Check sheet for the modelled part. Datum: model origin and axes. Units: mm. A direction names the side the tool comes from. Give positions to 0.01 mm unless a question says otherwise; leave off trailing zeros. Order: outer loops, then holes, each group sorted by start corner. A loop starts at its lowest first (then second) coordinate and runs counter-clockwise, first axis right, second up. Notation, with made-up numbers: M 89.25,24.5 L 100.25,24.5 A15 ccw 100.25,45.5 Z; hole C 87.5,-39.75 d9. An arc over 180 degrees is marked long. Return JSON: item names as keys, results as strings. Group by question number.
from build123d import *

# Parameters (mm, degrees)
SKETCH1_R           = 3
BOSS_EXTRUDE1_DEPTH = 3
CUT_EXTRUDE1_DEPTH  = 1.5
SKETCH4_R           = 1.35
BOSS_EXTRUDE2_DEPTH = 8.5


with BuildPart() as part:
    # Sketch1 → Boss-Extrude1 (new body)
    with BuildSketch(Plane.XY):
        Circle(SKETCH1_R)
    extrude(amount=BOSS_EXTRUDE1_DEPTH)

    # Sketch2 → Cut-Extrude1 (cut)
    with BuildSketch(Plane.XY.offset(3)):
        Polygon((2.06190779, 0), (1.030953895, 1.785664527), (-1.030953895, 1.785664527), (-2.06190779, 0), (-1.030953895, -1.785664527), (1.030953895, -1.785664527), align=None)
    extrude(amount=-CUT_EXTRUDE1_DEPTH, mode=Mode.SUBTRACT)

    # Sketch4 → Boss-Extrude2 (add)
    with BuildSketch(Plane(origin=(0, 0, 0), x_dir=(-1, 0, 0), z_dir=(0, 0, -1))):
        Circle(SKETCH4_R)
    extrude(amount=BOSS_EXTRUDE2_DEPTH)


solid = part.part
1) Sectioned sample at A-A on x = 0. Record the boundary of the cut face in (y, z).
2) Sectioned sample at B-B on y = 0.3. Record the boundary of the cut face in (x, z).
3) Sectioned sample at C-C on z = -3.25. Record the boundary of the cut face in (x, y).
4) Tool access check on faces 1 (the face through (0, -2, 3)), 2 (the face through (0, -1.786, 2)). Record the directions out of +Z, -Z, +X, -X, +Y, -Y that give a thin tool (end or side, any length) a straight path to the whole face; none if there is none.
5) Depth check by flat-ended pin: P1, Ø2, axis at x = -1.5, y = 2, coming from the -Z side; P2, Ø1.2, axis at x = -0.5, z = 2, coming from the -Y side; P3, Ø1, axis at y = 2, z = 1, coming from the -X side. Enter the tip coordinate at first touch or a pass-through.
6) Material ranges on line 1 along Z through (x, y) = (0.45, 0.4); line 2 along Z through (x, y) = (1.35, -1.65); line 3 along Y through (x, z) = (-0.65, -7.5), recorded low to high.
7) Release check for a two-part mould opening along Y. For faces 3 (the face through (0, 0, -8.5)), 4 (the face through (-1.539, 0.905, 2.26)), 5 (the face through (0.29, -1.32, -4.19)) record: released by +Y, released by -Y, zero draft, split by the parting line, or undercut.
8) Sectioned sample at D-D on x = -1.7. Record the boundary of the cut face in (y, z).
Reply:
{
 "1": {"outline": "M -3,0 L -1.35,0 L -1.35,-8.5 L 1.35,-8.5 L 1.35,0 L 3,0 L 3,3 L 1.79,3 L 1.79,1.5 L -1.79,1.5 L -1.79,3 L -3,3 Z"},
 "2": {"outline": "M -2.98,0 L -1.32,0 L -1.32,-8.5 L 1.32,-8.5 L 1.32,0 L 2.98,0 L 2.98,3 L 1.89,3 L 1.89,1.5 L -1.89,1.5 L -1.89,3 L -2.98,3 Z"},
 "3": {"outline": "C 0,0 d2.7"},
 "4": {"face 1": "+Z, +X, -X, +Y, -Y", "face 2": "+Z"},
 "5": {"P1": "z = 0", "P2": "y = -3", "P3": "x = -2.6"},
 "6": {"line 1": "-8.5 to 1.5", "line 2": "0 to 3", "line 3": "-1.18 to 1.18"},
 "7": {"face 3": "zero draft", "face 4": "undercut", "face 5": "split by the parting line"},
 "8": {"outline": "M -2.47,0 L 2.47,0 L 2.47,3 L 0.63,3 L 0.63,1.5 L -0.63,1.5 L -0.63,3 L -2.47,3 Z"}
}
